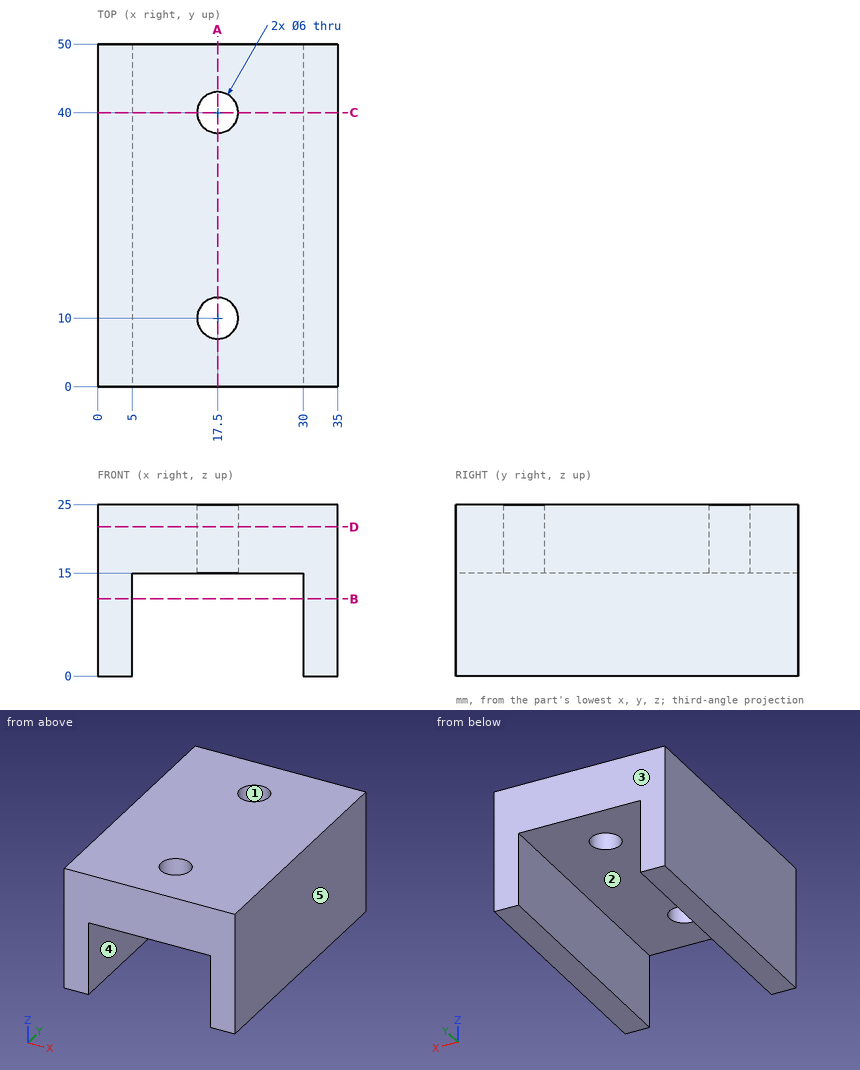
Check sheet for the drawn part. Datum: minimum x, y, z corner. Units: mm. A direction names the side the tool comes from. Round coordinates to 2 decimals unless told otherwise and drop trailing zeros. Loops run counter-clockwise (first coordinate to the right, second up) from the corner with the lowest first, then second, coordinate; pieces in that order, holes last. Notation, with made-up numbers: (77.5, 72.5) - (90.5, 72.5) arc R12 ccw to (90.5, 77.5) - close; hole circle Ø3 at (37.25, -16.75). An arc over 180 degrees is marked (long way). Write each question's results on one line, items separated by ' | '. Start each with the question number.
Q1. Cross-section at C-C on y = 40. Enter the section's corners in (x, z).
Q2. Access from +Z, -Z, +X, -X, +Y, -Y to the whole of each face (thin tool, end or side, straight path). Record for the marked faces 1 and 2.
Q3. Cross-section at B-B on z = 11.25. Enter the section's corners in (x, y), and give its area (3 significant figures).
Q4. Release check for a two-part mould opening along X. For the marked faces 3, 4 and 5 record: +X half, -X half, draft (parallel to the pull), parting line (faces both ways), or undercut.
Q5. Gauge pin test, flat end, axial feed: P1, Ø1, axis at x = 8, y = 28, coming from the -Z side. Record the tip position at first contact, or that the pin passes through.
Q6. Cross-section at A-A on x = 17.5. Enter the section's corners in (y, z).
Q7. Cross-section at D-D on z = 21.75. Enter the section's corners in (x, y), and give its area (3 significant figures).
Q8. Thickness scan on line 1 (Y direction, x = 17.5, z = 21); line 2 (X direction, y = 13, z = 12.5); line 3 (Z direction, x = 9, y = 16). Record the ranges inside material, lowest first. Write a range as [from, to].
Answers below:
1) outline: (0, 0) - (5, 0) - (5, 15) - (14.5, 15) - (14.5, 25) - (0, 25) - close; (20.5, 15) - (30, 15) - (30, 0) - (35, 0) - (35, 25) - (20.5, 25) - close
2) face 1: +Z, -Z | face 2: -Z, +Y, -Y
3) outline: (0, 0) - (5, 0) - (5, 50) - (0, 50) - close; (30, 0) - (35, 0) - (35, 50) - (30, 50) - close | area: 500 mm²
4) face 3: draft | face 4: undercut | face 5: +X half
5) P1: stops at z = 15
6) outline: (0, 15) - (7, 15) - (7, 25) - (0, 25) - close; (13, 15) - (37, 15) - (37, 25) - (13, 25) - close; (43, 15) - (50, 15) - (50, 25) - (43, 25) - close
7) outline: (0, 0) - (35, 0) - (35, 50) - (0, 50) - close; hole circle Ø6 at (17.5, 10); hole circle Ø6 at (17.5, 40) | area: 1,690 mm²
8) line 1: y = [0, 7], [13, 37], [43, 50] | line 2: x = [0, 5], [30, 35] | line 3: z = [15, 25]
